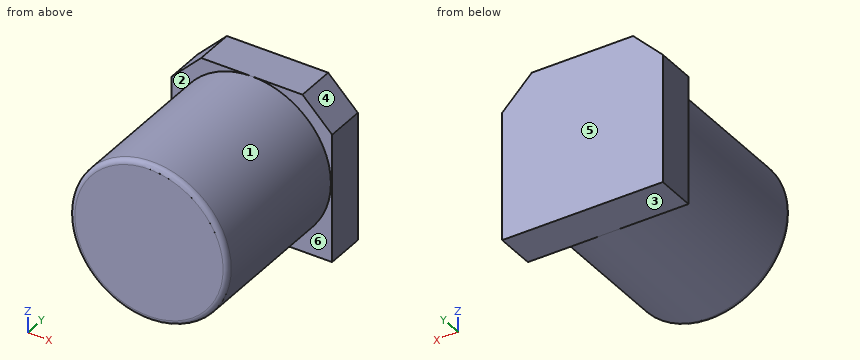
from build123d import *

# Parameters (mm, degrees)
F0_R     = 3.175
F1_DEPTH = 6.35
F3_DEPTH = 1.5875
F4_R     = 0.1984375


with BuildPart() as f1:
    # F0 (on Front) → F1 (new body)
    with BuildSketch(Plane.XZ):
        Circle(F0_R)
    extrude(amount=F1_DEPTH)

    # F2 (on face) → F3 (join)
    with BuildSketch(Plane(origin=(0, 0, 0), x_dir=(-1, 0, 0), z_dir=(0, 1, 0))):
        with BuildLine():
            Line((0, 3.175), (-2.033528515, 3.175))
            Line((-2.033528515, 3.175), (-3.224153515, 1.984375))
            Line((-3.224153515, 1.984375), (-3.224153515, -3.175))
            Line((-3.224153515, -3.175), (0, -3.175))
            ThreePointArc((0, -3.175), (-3.175, 0), (0, 3.175))
        make_face()
        with BuildLine():
            Line((2.033528515, 3.175), (0, 3.175))
            ThreePointArc((0, 3.175), (2.2450640303, 2.2450640303), (3.175, 0))
            ThreePointArc((3.175, 0), (2.2450640303, -2.2450640303), (0, -3.175))
            Line((0, -3.175), (3.224153515, -3.175))
            Line((3.224153515, -3.175), (3.224153515, 1.984375))
            Line((3.224153515, 1.984375), (2.033528515, 3.175))
        make_face()
        with BuildLine():
            ThreePointArc((3.175, 0), (2.2450640303, 2.2450640303), (0, 3.175))
            ThreePointArc((0, 3.175), (-3.175, 0), (0, -3.175))
            ThreePointArc((0, -3.175), (2.2450640303, -2.2450640303), (3.175, 0))
        make_face()
    extrude(amount=F3_DEPTH)

    # F4
    f4_edges = [f1.edges().sort_by_distance(p)[0] for p in [
        (-3.175, -6.35, 0),
    ]]
    fillet(f4_edges, radius=F4_R)


solid = f1.part
Build history of the part. All positions in model axes, mm. Face numbers are marked on the shaded views. A direction names the side the tool comes from. Coordinates: 2 decimals unless noted, no trailing zeros. Order: outer loops, then holes, each group sorted by start corner. A loop starts at its lowest first (then second) coordinate and runs counter-clockwise, first axis right, second up. Notation, with made-up numbers: (77, -6.75) -> (99, -6.75) arc R27 cw to (99, 26.25) -> close; hole circle Ø8 at (33, -29.75). An arc over 180 degrees is marked (long way). One line per item, written item: value.
(1) Probe line 1 (Y direction, x = -2.5, z = 2); line 2 (Y direction, x = 2.25, z = 2); line 3 (Z direction, x = 1, y = -1.5). List the from-to ranges inside material, lowest first. Write a range as [from, to].
Checked values:
line 1: [0, 1.59]
line 2: [-6.35, 1.59]
line 3: [-3.01, 3.01]
(2) Mould opens along Y. For the marked faces 4, 5 and 6 say: pulls with the +Y half, pulls with the -Y half, needs draft (parallel to the pull), parting line crosses it, or undercut.
Checked values:
face 4: needs draft
face 5: pulls with the +Y half
face 6: pulls with the -Y half
(3) Drop a flat-ended pin along its axis: pin 1 Ø2 at (x, y) = (-2, -3.5) entering from -Z. Give the stop position or say it passes through.
Checked values:
pin 1: z = -3.01
(4) Slice it at B-B, the plane y = -4. List the corners of the cut face in (x, z) (3 decimals), plus the area to 3 significant figures.
Checked values:
outline: circle Ø6.35 at (0, 0)
area: 31.7 mm2
(5) Slice it at A-A, the plane y = 1. List the corners of the cut face in (x, z) (3 decimals).
Checked values:
outline: (-3.224, -3.175) -> (3.224, -3.175) -> (3.224, 1.984) -> (2.034, 3.175) -> (-2.034, 3.175) -> (-3.224, 1.984) -> close
(6) Tool access for the marked faces 1, 2 and 3: list every direction of +Z, -Z, +X, -X, +Y, -Y with a clear straight run to the whole face (end or side of a thin tool).
Checked values:
face 1: -Y
face 2: -X, -Y
face 3: -Z, +X, -X, +Y, -Y
